Input: part model. Units: mm. Frame: model coordinates. A direction names the side the tool comes from. Round coordinates to 2 decimals unless told otherwise and drop trailing zeros. Loops run counter-clockwise (first coordinate to the right, second up) from the corner with the lowest first, then second, coordinate; pieces in that order, holes last. Notation, with made-up numbers: (-11, 78.25) - (21, 78.25) arc R10 cw to (21, 83.25) - close; hole circle Ø10 at (-33.5, 15). An arc over 180 degrees is marked (long way). Use CSV: the item, a comma, the result in double quotes. Start each with the question number.
1. Pin query (flat end, axial travel): P1, Ø10, axis at x = 1.5, z = 10.5, coming from the -Y side; P2, Ø3, axis at x = 35, z = 56, coming from the -Y side; P3, Ø1.5, axis at y = 6.5, z = 70.5, coming from the -X side. Return the tip coordinate at first contact, or that it passes through.
2. Material intervals for probe 1 along Y at (x, z) = (-8, 63.5); probe 2 along Z at (x, y) = (38, -9.5); probe 3 along Z at (x, y) = (5.5, 2), sorted ascending. Write a range as from..to.
3. Cut plane C-C (x = -24). Return loops of the section in (y, z), and give its area (3 significant figures).
4. Access query for faces 1 (the flat face through (-23.187, -13.827, 10.273)), 2 (the flat face through (13, -18, 38.1)), 3 (the flat face through (-2, 8, 78.74)). Directions: +Z, -Z, +X, -X, +Y, -Y. A direction counts if a zero-diameter tool reaches every point of the face in a straight line with its end or side. Return the directions, or none.
5. Pull-direction query (X, two-part tool) for faces 4 (the flat face through (-3, -3, 20.263)), 5 (the flat face through (1, 2.099, 58)), 6 (the flat face through (-53.732, -13, 24)), 7 (the flat face through (44.683, 8.225, 71.765)); classes: +X half, -X half, draft (parallel to the pull), parting line (faces both ways), or undercut.
6. Cut plane A-A (y = -6.5). Return loops of the section in (x, z).
7. Cut plane D-D (z = 56). Return loops of the section in (x, y).
8. Cut plane B-B (z = 24). Return loops of the section in (x, y), and give its area (3 significant figures).
```python
from build123d import *

# Parameters (mm, degrees)
F0_W      = 110.8218282461
F0_H      = 53.3959735185
F1_DEPTH  = 38.1
F2_W      = 110.8218282461
F2_H      = 12.4254778493
F3_DEPTH  = 40.64
F5_DEPTH  = 25.4
F7_DEPTH  = 25.4
F8_DEPTH  = 25.4
F10_DEPTH = 25.4


with BuildPart() as f1:
    # F0 (on Top) → F1 (new body)
    with BuildSketch(Plane.XY):
        with Locations((1.6791187227, -12.1736107394)):
            Rectangle(F0_W, F0_H)
    extrude(amount=F1_DEPTH)

    # F2 (on face) → F3 (join)
    with BuildSketch(Plane.XY.offset(38.1)):
        with Locations((1.6791187227, 8.3116370952)):
            Rectangle(F2_W, F2_H)
    extrude(amount=F3_DEPTH)

    # F4 (on face) → F5 (cut)
    with BuildSketch(Plane.XZ.offset(-2.0988981705)):
        Polygon((-53.7317954004, 62.9949569702), (-35.2727063, 78.74), (-53.7317954004, 78.74), align=None)
        Polygon((57.0900328457, 78.74), (32.6191671193, 78.74), (57.0900328457, 64.5924061537), align=None)
    extrude(amount=-F5_DEPTH, mode=Mode.SUBTRACT)

    # F6 (on face) → F7 (cut)
    with BuildSketch(Plane.XZ.offset(38.8715974987)):
        Polygon((-29.8812910914, 20.2630087733), (-16.3029171526, 0), (13.250015676, 0), (24.0328423679, 20.2630087733), align=None)
    extrude(amount=-F7_DEPTH, mode=Mode.SUBTRACT)

    # F8 (cut): a face of the model
    f8_faces = [f1.faces().sort_by_distance(p)[0] for p in [
        (-2.2933313213, -13.4715974987, 11.1171850151),
    ]]
    extrude(f8_faces, amount=-F8_DEPTH, mode=Mode.SUBTRACT)

    # F9 (on face) → F10 (cut)
    with BuildSketch(Plane.XY.offset(38.1)):
        with BuildLine():
            Line((-12.7204942497, -17.3120461404), (0, -17.3120461404))
            Line((0, -17.3120461404), (0, -4.5915518908))
            ThreePointArc((0, -4.5915518908), (-8.994747744, -8.3172983965), (-12.7204942497, -17.3120461404))
        make_face()
        with BuildLine():
            Line((0, -4.5915518908), (0, -17.3120461404))
            Line((0, -17.3120461404), (12.7204942497, -17.3120461404))
            ThreePointArc((12.7204942497, -17.3120461404), (8.994747744, -8.3172983965), (0, -4.5915518908))
        make_face()
        with BuildLine():
            Line((0, -30.0325403901), (0, -17.3120461404))
            Line((0, -17.3120461404), (-12.7204942497, -17.3120461404))
            ThreePointArc((-12.7204942497, -17.3120461404), (-8.994747744, -26.3067938844), (0, -30.0325403901))
        make_face()
        with BuildLine():
            Line((12.7204942497, -17.3120461404), (0, -17.3120461404))
            Line((0, -17.3120461404), (0, -30.0325403901))
            ThreePointArc((0, -30.0325403901), (8.994747744, -26.3067938844), (12.7204942497, -17.3120461404))
        make_face()
    extrude(amount=-F10_DEPTH, mode=Mode.SUBTRACT)


solid = f1.part
```
Established:
1,P1,"stops at y = 11.93"
1,P2,"stops at y = 2.1"
1,P3,"stops at x = -45.81"
2,probe 1,"y = 2.1..14.52"
2,probe 2,"z = 0..38.1"
2,probe 3,"z = 20.26..38.1"
3,outline,"(-38.87, 0) - (14.52, 0) - (14.52, 78.74) - (2.1, 78.74) - (2.1, 38.1) - (-38.87, 38.1) - (-38.87, 20.26) - (11.93, 20.26) - (11.93, 11.49) - (-38.87, 11.49) - close"
3,area,"2,090 mm2"
4,face 1,"-Y"
4,face 2,"+Z, +X, -X, -Y"
4,face 3,"+Z, +X, -X, +Y, -Y"
5,face 4,"undercut"
5,face 5,"draft"
5,face 6,"-X half"
5,face 7,"+X half"
6,outline,"(-53.73, 0) - (-16.3, 0) - (-29.88, 20.26) - (-6.7, 20.26) - (-6.7, 38.1) - (-53.73, 38.1) - close; (6.7, 20.26) - (24.03, 20.26) - (13.25, 0) - (57.09, 0) - (57.09, 38.1) - (6.7, 38.1) - close"
7,outline,"(-53.73, 2.1) - (57.09, 2.1) - (57.09, 14.52) - (-53.73, 14.52) - close"
8,outline,"(-53.73, -38.87) - (57.09, -38.87) - (57.09, 14.52) - (-53.73, 14.52) - close; hole circle Ø25.44 at (0, -17.31)"
8,area,"5,410 mm2"
